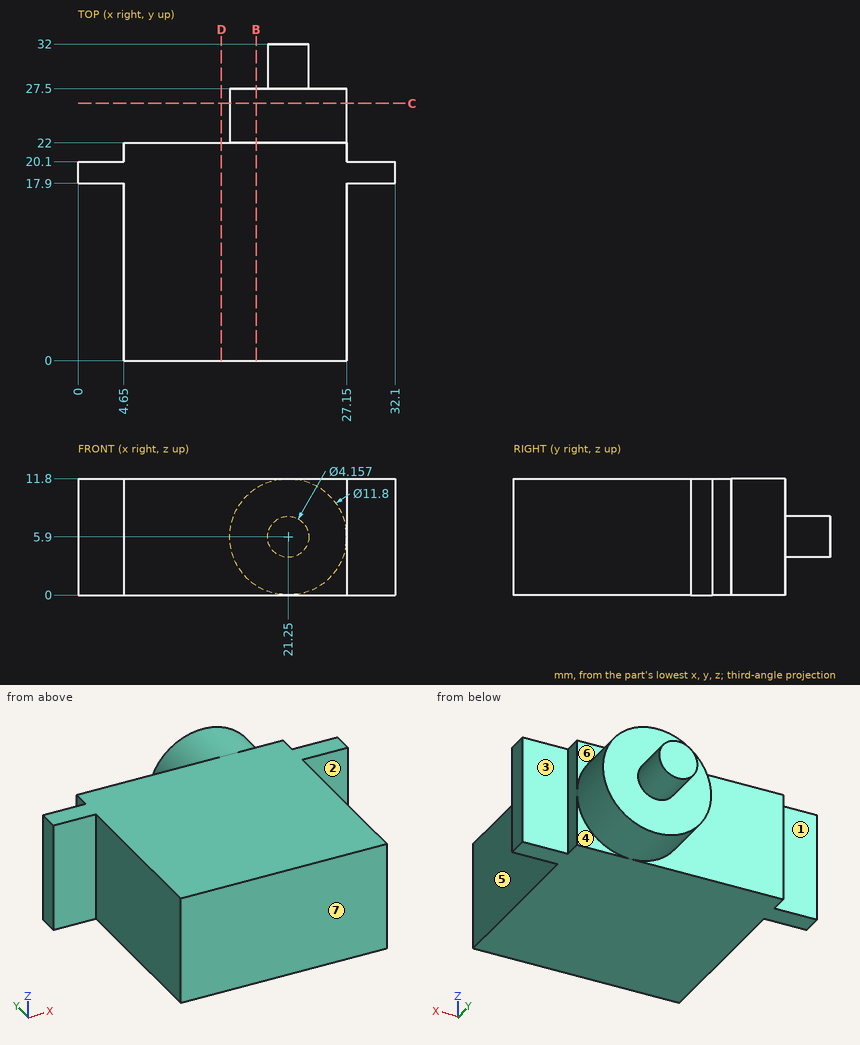
Here's the drawing with two shaded views (mm, measured from the low corner). I have some questions. A direction names the side the tool comes from. Round coordinates to 2 decimals unless told otherwise and drop trailing zeros. Write each loop counter-clockwise with the first axis right and the second up, starting at its lowest first coordinate (ties: lowest second). Pieces come first, ordered by that corner, then holes. Notation, with made-up numbers: M -16.75,67 L 30.25,67 A10 ccw 30.25,84 Z; hole C 67.5,-7 d7. An arc over 180 degrees is marked long. Answer in a Markdown table with one row per item. Add a question column.
Q1. Will these pins go through, and if not, where does the flat tip stop? pin 1 Ø1.5 at (x, z) = (30.5, 5.5) entering from +Y; pin 2 Ø5 at (y, z) = (15, 8) entering from +X; pin 3 Ø1.8 at (x, z) = (24, 9) entering from +Y.
Q2. Imagine slicing it at B-B (x = 18). Please give me the cut outline in (y, z) (1 decimal), then the cut area to 3 significant figures.
Q3. Imagine slicing it at C-C (y = 26). Please give me the cut outline in (x, z), then the cut area to 3 significant figures.
Q4. If we mould it in two halves opening along Y, with no side actions, what happens to the marked faces 5, 6 and 7? For each: +Y half, -Y half, draft (parallel to the pull), parting line (faces both ways), or undercut.
Q5. Imagine slicing it at D-D (x = 14.5). Please give me the cut outline in (y, z).
Q6. On a 3-axis mill with a long thin cutter (end or side, diameter ignored), from which of +Z, -Z, +X, -X, +Y, -Y can I reach the whole of each face in a straight line? I mean the marked faces 1, 2, 3 and 4. Say none if no direction works.
Q7. If I drill on line 1 (Y direction, x = 17, z = 5.5); line 2 (X direction, y = 2, z = 2.25); line 3 (Y direction, x = 6, z = 3.25), over which ranges is the centre line in solid material (lowest first)? Write a range as from..to.
Values:
| question | item | result |
|---|---|---|
| 1 | pin 1 | y = 20.1 |
| 1 | pin 2 | x = 27.15 |
| 1 | pin 3 | y = 27.5 |
| 2 | outline | M 0,0 L 22,0 L 22,1 L 27.5,1 L 27.5,10.8 L 22,10.8 L 22,11.8 L 0,11.8 Z |
| 2 | area | 314 mm^2 |
| 3 | outline | C 21.25,5.9 d11.8 |
| 3 | area | 109 mm^2 |
| 4 | face 5 | draft |
| 4 | face 6 | +Y half |
| 4 | face 7 | -Y half |
| 5 | outline | M 0,0 L 22,0 L 22,11.8 L 0,11.8 Z |
| 6 | face 1 | +Z, -Z, -X, +Y |
| 6 | face 2 | +Z, -Z, +X, -Y |
| 6 | face 3 | +Z, -Z, +X, +Y |
| 6 | face 4 | -Z, +X, +Y |
| 7 | line 1 | 0..27.5 |
| 7 | line 2 | 4.65..27.15 |
| 7 | line 3 | 0..22 |
